Autodesk Inventor part; units mm, degrees
ref_plane "YZ Plane" through (0, 0, 0) normal (1, 0, 0) x (0, 1, 0)
ref_plane "XZ Plane" through (0, 0, 0) normal (0, 1, 0) x (-1, 0, 0)
ref_plane "XY Plane" through (0, 0, 0) normal (0, 0, 1) x (1, 0, 0)
sketch "Sketch1" plane through (0, 0, 0) normal (0, 1, 0) x (-1, 0, 0)
  circle A0 centre (0, 0) radius 30
  dimension "d0" = 60
extrude "Extrusion1" add sketch "Sketch1" along normal mid plane 270
sketch "Sketch2" plane through (0, -135, 0) normal (0, -1, 0) x (1, 0, 0)
  circle A0 centre (0, 0) radius 8.5
  dimension "d3" = 17
extrude "Extrusion2" add sketch "Sketch2" along normal blind 30
sketch "Sketch3" plane through (0, 135, 0) normal (0, 1, 0) x (1, 0, 0)
  circle A0 centre (0, 0) radius 8.5
  circle A1 centre (0, 0) radius 8.5
  dimension "d6" = 17
extrude "Extrusion3" add sketch "Sketch3" along normal blind 100
sketch "Sketch4" plane through (0, 235, 0) normal (0, 1, 0) x (1, 0, 0)
  circle A0 centre (0, 0) radius 8.5
  circle A1 centre (0, 0) radius 6
  dimension "d9" = 12
extrude "Extrusion4" cut sketch "Sketch4" against normal blind 60
properties part number "HCMUTE-CDT23-TRUC_DAN" material "Stainless Steel"
Could you check a few things on this model? Use its own coordinates, in mm. A direction names the side the tool comes from. Coordinates: 2 decimals unless noted, no trailing zeros. Order: outer loops, then holes, each group sorted by start corner. A loop starts at its lowest first (then second) coordinate and runs counter-clockwise, first axis right, second up.
Q1. Suppose I cut it at C-C on y = 6. Please give me the cut outline in (x, z), and give its area (3 significant figures).
Q2. Which directions (+Z, -Z, +X, -X, +Y, -Y) give clear straight access to the entire face, cutting with the end or side of a thin tool? Please do faces 1 (the flat face through (-6.2, -135, -6.2)), 2 (the cylindrical face through (29.97, -1.89, -1.32)), 3 (the flat face through (2, 175, -6)).
Q3. Suppose I cut it at D-D on y = 164.5. Please give me the cut outline in (x, z).
Q4. Suppose I cut it at A-A on z = 0. Please give me the cut outline in (x, y), and give its area (3 significant figures).
Q5. Suppose I cut it at B-B on x = 0. Please give me the cut outline in (y, z), and give its area (3 significant figures).
Q6. Please list where these lines run through material, in increasing order: L1, parallel to Y at x = 10, z = -9; L2, parallel to Y at x = -8, z = -1; L3, parallel to Z at x = 2, y = 108.
Q7. Will these pins go through, and if not, where does the flat tip stop? pin 1 (1 mm diameter, centred on y = 20.5, z = -22, fed in from +X); pin 2 (2 mm diameter, centred on x = -0.5, z = 14, fed in from -Y); pin 3 (8 mm diameter, centred on y = -1.5, z = -0.5, fed in from -X); pin 4 (1.5 mm diameter, centred on x = -6, z = 20.5, fed in from +Y).
Answer:
1. outline: circle Ø60 at (0, 0)
1. area: 2,830 mm2
2. face 1: -Y
2. face 2: +Y, -Y
2. face 3: +Y
3. outline: circle Ø17 at (0, 0)
4. outline: (-30, -135) - (-8.5, -135) - (-8.5, -165) - (8.5, -165) - (8.5, -135) - (30, -135) - (30, 135) - (8.5, 135) - (8.5, 175) - (6, 175) - (6, 235) - (-6, 235) - (-6, 175) - (-8.5, 175) - (-8.5, 135) - (-30, 135) - close
4. area: 18,100 mm2
5. outline: (-165, -8.5) - (-135, -8.5) - (-135, -30) - (135, -30) - (135, -8.5) - (175, -8.5) - (175, -6) - (235, -6) - (235, 6) - (175, 6) - (175, 8.5) - (135, 8.5) - (135, 30) - (-135, 30) - (-135, 8.5) - (-165, 8.5) - close
5. area: 18,100 mm2
6. L1: y = -135 to 135
6. L2: y = -165 to 175
6. L3: z = -29.93 to 29.93
7. pin 1: stops at x = 20.92
7. pin 2: stops at y = -135
7. pin 3: stops at x = -30
7. pin 4: stops at y = 135
